Part model, mm, in its own coordinate system. Face numbers are marked on the shaded views. A direction names the side the tool comes from. Round coordinates to 2 decimals unless told otherwise and drop trailing zeros. Write each loop counter-clockwise with the first axis right and the second up, starting at its lowest first coordinate (ties: lowest second). Pieces come first, ordered by that corner, then holes.
1) Pull direction X, two halves, no side cores. Call the marked faces 3, 4 and 5: +X half, -X half, draft (parallel to the pull), parting line (faces both ways), or undercut.
2) Saw through at A-A on y = 8. Write the cut outline in (x, z).
3) Saw through at C-C on z = 2. Write the cut outline in (x, y).
4) Saw through at B-B on z = 6. Write the cut outline in (x, y), and give its area (3 significant figures).
5) Saw through at D-D on x = 0. Write the cut outline in (y, z).
6) Flat gauge pins, fed straight in: pin 1 (2.5 mm diameter, centred on y = -35, z = 5, fed in from +X); pin 2 (2.5 mm diameter, centred on x = -25.5, z = 3, fed in from -Y); pin 3 (8 mm diameter, centred on y = -33.5, z = 4.5, fed in from +X); pin 4 (3 mm diameter, centred on x = 26.5, z = 16.5, fed in from +Y). Where does each tip first touch, or does it go through?
7) Which spindle directions (+Z, -Z, +X, -X, +Y, -Y) get a long thin tool onto all of the face, cutting with end or side? Do the marked faces 1 and 2. Say none if no direction does.
8) Drill centre lines: L1, parallel to Z at x = 25, y = 4; L2, parallel to X at y = -36.5, z = 8; L3, parallel to Z at x = -21, y = -35. Where is each one in solid material? Low to high.
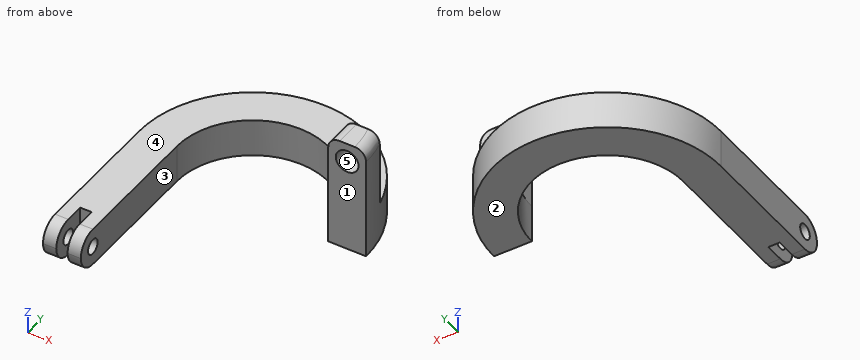
```python
from build123d import *

# Parameters (mm, degrees)
F1_DEPTH = 10
F2_R     = 4.99999
F3_R     = 2
F4_DEPTH = 25
F6_DEPTH = 30
F7_R     = 3
F8_R     = 3
F9_DEPTH = 25


# Not quite as in the source:
# - a fillet or chamfer is up to 0.001 mm smaller than in the source, because OpenCascade refuses the exact size


with BuildPart() as f1:
    # F0 (on Top) → F1 (new body)
    with BuildSketch(Plane.XY):
        with BuildLine():
            ThreePointArc((-20, 0), (0, 20), (20, 0))
            Line((20, 0), (30, 0))
            ThreePointArc((30, 0), (0, 30), (-30, 0))
            Line((-30, 0), (-30, -40))
            Line((-30, -40), (-26.5, -40))
            Line((-26.5, -40), (-26.5, -30))
            Line((-26.5, -30), (-23.5, -30))
            Line((-23.5, -30), (-23.5, -40))
            Line((-23.5, -40), (-20, -40))
            Line((-20, -40), (-20, 0))
        make_face()
    extrude(amount=F1_DEPTH)

    # F2 (radius 5 in the source; OpenCascade refuses exactly that, so slightly less here)
    f2_edges = [f1.edges().sort_by_distance(p)[0] for p in [
        (-28.25, -40, 10),
        (-28.25, -40, 0),
        (-21.75, -40, 10),
        (-21.75, -40, 0),
    ]]
    fillet(f2_edges, radius=F2_R)

    # F3 (on face) → F4 (cut)
    with BuildSketch(Plane.YZ.offset(-20)):
        with Locations((-35, 5)):
            Circle(F3_R)
    extrude(amount=-F4_DEPTH, mode=Mode.SUBTRACT)

    # F5 (on face) → F6 (join)
    with BuildSketch(Plane(origin=(0, 0, 0), x_dir=(1, 0, 0), z_dir=(0, 0, -1))):
        with BuildLine():
            ThreePointArc((29.1719042916, -7), (29.7922567855, -3.5244057124), (30, 0))
            Line((30, 0), (20, 0))
            Line((20, 0), (20, -7))
            Line((20, -7), (29.1719042916, -7))
        make_face()
    extrude(amount=-F6_DEPTH)

    # F7
    f7_edges = [f1.edges().sort_by_distance(p)[0] for p in [
        (29.792257, 3.524406, 30),
        (20, 3.5, 30),
    ]]
    fillet(f7_edges, radius=F7_R)

    # F8 (on face) → F9 (cut)
    with BuildSketch(Plane(origin=(0, 7, 0), x_dir=(-1, 0, 0), z_dir=(0, 1, 0))):
        with Locations((-25, 25)):
            Circle(F8_R)
    extrude(amount=-F9_DEPTH, mode=Mode.SUBTRACT)


solid = f1.part
```
Completed:
1. face 3: +X half
1. face 4: draft
1. face 5: undercut
2. outline: (-28.91, 0) - (-18.33, 0) - (-18.33, 10) - (-28.91, 10) - close; (18.33, 0) - (28.91, 0) - (28.91, 10) - (18.33, 10) - close
3. outline: (-30, -39) - (-26.5, -39) - (-26.5, -30) - (-23.5, -30) - (-23.5, -39) - (-20, -39) - (-20, 0) arc R20 cw to (20, 0) - (30, 0) arc R30 ccw to (-30, 0) - close
4. outline: (-30, -39.9) - (-26.5, -39.9) - (-26.5, -36.73) - (-30, -36.73) - close; (-30, -33.27) - (-26.5, -33.27) - (-26.5, -30) - (-23.5, -30) - (-23.5, -33.27) - (-20, -33.27) - (-20, 0) arc R20 cw to (20, 0) - (30, 0) arc R30 ccw to (-30, 0) - close; (-23.5, -39.9) - (-20, -39.9) - (-20, -36.73) - (-23.5, -36.73) - close
4. area: 1,130 mm2
5. outline: (20, 0) - (30, 0) - (30, 10) - (20, 10) - close
6. pin 1: passes through
6. pin 2: stops at y = -39.84
6. pin 3: stops at x = -20
6. pin 4: stops at y = 7
7. face 1: +Z, -Z, +X, -Y
7. face 2: -Z, +X, -X, +Y, -Y
8. L1: z = 0 to 22, 28 to 30
8. L2: x = -30 to -26.5, -23.5 to -20
8. L3: z = 0 to 3, 7 to 10
